For this review, take the finished solid that the model builds, in its own axes (mm). A direction names the side the tool comes from. Coordinates: 2 decimals unless noted, no trailing zeros. Write each loop counter-clockwise with the first axis right and the second up, starting at its lowest first coordinate (ties: lowest second). Pieces come first, ordered by that corner, then holes. Notation, with made-up numbers: M 66.5,69 L 93.5,69 A32 ccw 93.5,108 Z; hole C 67,7.5 d10. An arc over 180 degrees is marked long. Return JSON: item names as keys, results as strings.
```python
from build123d import *

# Parameters (mm, degrees)
F0_W        = 23.8125
F0_H        = 12.5
F1_DEPTH    = 10
F2_W        = 9.5
F2_H        = 8.5
F3_DEPTH    = 23.8135
F4_W        = 11.5
F4_H        = 12.5
F5_DEPTH    = 20
F6_SIZE2    = 18
F6_SIZE     = 10
F7_T4_DEPTH = 48.8797731496
F7_T9_DEPTH = 48.8797731496
F8_W        = 2
F8_H        = 3.4425717247


# Not quite as in the source:
# - a fillet or chamfer that OpenCascade refuses, or shapes differently, is made with other operations: its cross-section is extruded or revolved along the edge and cut away or added


with BuildPart() as f1:
    # F0 (on Top) → F1 (new body)
    with BuildSketch(Plane.XY):
        with Locations((-12.5924281826, 6.2716105528)):
            Rectangle(F0_W, F0_H)
    extrude(amount=F1_DEPTH)

    # F2 (on face) → F3 (cut, through all)
    with BuildSketch(Plane.YZ.offset(-0.6861781826)):
        with Locations((6.2716105528, 4.25)):
            Rectangle(F2_W, F2_H)
    extrude(amount=-F3_DEPTH, mode=Mode.SUBTRACT)

    # F4 (on face) → F5 (join)
    with BuildSketch(Plane.XY.offset(10)):
        with Locations((-6.4361781826, 6.2716105528)):
            Rectangle(F4_W, F4_H)
    extrude(amount=F5_DEPTH)

    # F6
    f6_edges = [f1.edges().sort_by_distance(p)[0] for p in [
        (-12.186178, 6.271611, 30),
    ]]
    f6_side = f1.faces().sort_by_distance((-6.436178, 6.271611, 30))[0]
    chamfer(f6_edges, length=F6_SIZE, length2=F6_SIZE2, reference=f6_side)

    # F7: chamfer of 5.5 on 2 edges, made by hand


with BuildPart() as f7_tool2:
    # F7_s3 → F7_t4 (new body)
    with BuildSketch(Plane(origin=(19.0892991485, 0, 34.3607384673), x_dir=(0, 1, 0), z_dir=(-0.4856429312, 0, -0.8741572761))):
        Polygon((12.5216105528, -10.9803515006), (7.0216105528, -16.4803515006), (12.5216105528, -16.4803515006), align=None)
    extrude(amount=F7_T4_DEPTH)

    split(bisect_by=Plane.XY.offset(10), keep=Keep.TOP)


with BuildPart() as f1_1:
    add(f1.part)

    # F7_t1: cut F7_tool2
    add(f7_tool2.part, mode=Mode.SUBTRACT)


with BuildPart() as f7_tool7:
    # F7_s8 → F7_t9 (new body)
    with BuildSketch(Plane(origin=(19.0892991485, 0, 34.3607384673), x_dir=(0, 1, 0), z_dir=(-0.4856429312, 0, -0.8741572761))):
        Polygon((5.5216105528, -16.4803515006), (0.0216105528, -10.9803515006), (0.0216105528, -16.4803515006), align=None)
    extrude(amount=F7_T9_DEPTH)

    split(bisect_by=Plane.XY.offset(10), keep=Keep.TOP)


with BuildPart() as f1_2:
    add(f1_1.part)

    # F7_t6: cut F7_tool7
    add(f7_tool7.part, mode=Mode.SUBTRACT)

    # F8 (on face) → F9 (revolve, cut)
    with BuildSketch(Plane.XY.offset(10)):
        with Locations((-11.1861781826, 6.2716105528)):
            Rectangle(F8_W, F8_H)
    revolve(axis=Axis((-12.1861781826, 6.2716105528, 10), (0, -1, 0)), mode=Mode.SUBTRACT)


solid = f1_2.part
```
1. Wall thickness on L1, parallel to Y at x = -6.5, z = 2; L2, parallel to Z at x = -18, y = 9.5; L3, parallel to Z at x = -6.25, y = 5.5: over which ranges is each line inside the solid? List them lowest first. Write a range as from..to.
Checks:
{"L1": "0.02..1.52, 11.02..12.52", "L2": "8.5..10", "L3": "8.5..22.64"}
2. We need section D-D (z = 12.5). State the section outline as (x, y) points.
Checks:
{"outline": "M -11.91,5.52 L -5.62,0.02 L -0.69,0.02 L -0.69,12.52 L -5.62,12.52 L -11.91,7.02 Z"}
3. For faces 1 (the face through (-14.014, 6.296, 9.188)), 2 (the face through (-1, 6, 30)), 3 (the face through (-13, 1, 0)), 4 (the face through (-12, 11.022, 4)), 5 (the face through (-11.7, 4.55, 9.8)), list the 3-axis set-ups (+Z, -Z, +X, -X, +Y, -Y) from which the entire face can be reached by the end or side of a thin tool; tool diameter is ignored.
Checks:
{"face 1": "+Z", "face 2": "+Z, +X, -X, +Y, -Y", "face 3": "-Z, +X, -X, +Y, -Y", "face 4": "-Z, +X, -X", "face 5": "none"}
4. We need section A-A (z = 5.5). State the section outline as (x, y) points.
Checks:
{"outline": "M -24.5,0.02 L -0.69,0.02 L -0.69,1.52 L -24.5,1.52 Z; M -24.5,11.02 L -0.69,11.02 L -0.69,12.52 L -24.5,12.52 Z"}
5. We need section C-C (y = 11.75). State the section outline as (x, z) points, plus the area to 3 significant figures.
Checks:
{"outline": "M -24.5,0 L -0.69,0 L -0.69,22.96 L -7.89,10 L -24.5,10 Z", "area": "285 mm2"}
6. We need section B-B (x = -15.25). State the section outline as (y, z) points.
Checks:
{"outline": "M 0.02,0 L 1.52,0 L 1.52,8.5 L 11.02,8.5 L 11.02,0 L 12.52,0 L 12.52,10 L 0.02,10 Z"}
7. Clearance check with flat-ended pins moving along their axes: pin 1 Ø10 at (x, z) = (-14.5, 16.5) entering from +Y; pin 2 Ø4 at (x, y) = (-13, 5) entering from +Z; pin 3 Ø3 at (y, z) = (11, 20.5) entering from -X. State where each tip first meets the part, or that it passes through.
Checks:
{"pin 1": "y = 7.81", "pin 2": "z = 14.01", "pin 3": "x = -4.82"}
8. Draft analysis for pull direction Z (two halves, no side actions). For faces 6 (the face through (-12.4, 8.3, 8.5)), 7 (the face through (-10.304, 6.296, 10.675)), 8 (the face through (-18, 6, 10)), state which applies: +Z half, -Z half, draft (parallel to the pull), parting line (faces both ways), or undercut.
Checks:
{"face 6": "-Z half", "face 7": "undercut", "face 8": "+Z half"}
